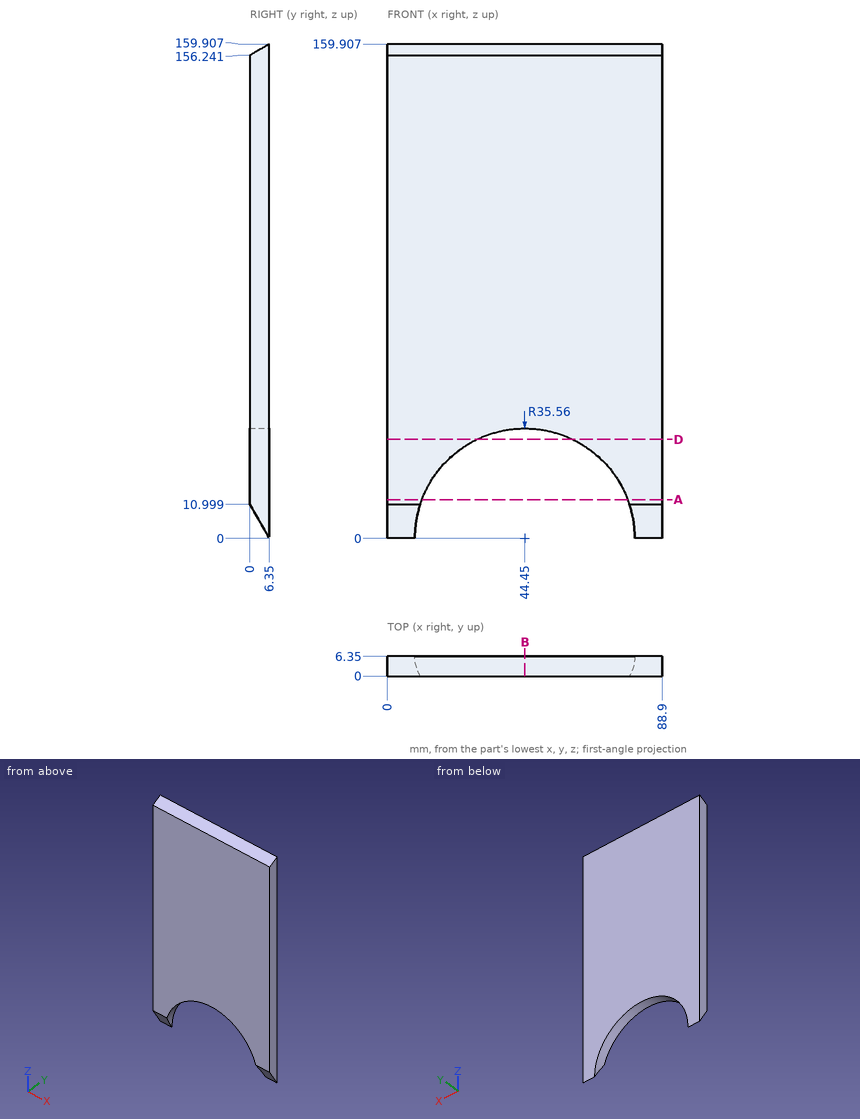
Verification items for this drawing (mm, ordinates from the low corner). Give positions to 0.01 mm unless a question says otherwise; leave off trailing zeros. Loops run counter-clockwise (first coordinate to the right, second up) from the corner with the lowest first, then second, coordinate; pieces in that order, holes last. Notation, with made-up numbers: M 39.5,41.25 L 43.5,41.25 A17 ccw 43.5,65.25 Z; hole C 0.5,12 d4. An arc over 180 degrees is marked long. Answer as a JSON object with one key per item and string values. Group by question number.
Q1. Cross-section at D-D on z = 32. Record the cut outline in (x, y).
Q2. Material ranges on line 1 along X through (y, z) = (3, 29); line 2 along X through (y, z) = (3, 29.5) (1 decimal); line 3 along Z through (x, y) = (65, 5.75), recorded low to high. Write a range as [from, to].
Q3. Go/stop test with flat-tipped pins: P1, Ø2, axis at x = 70, y = 4, coming from the +Z side; P2, Ø3, axis at x = 29, y = 4.5, coming from the +Z side (1 decimal); P3, Ø2, axis at x = 32, y = 5, coming from the -Z side; P4, Ø5, axis at x = 28.5, z = 29, coming from the +Y side. Record where each tip stops, or that it passes through.
Q4. Cross-section at B-B on x = 44.45. Record the cut outline in (y, z).
Q5. Cross-section at A-A on z = 12.5. Record the cut outline in (x, y).
Evaluation:
{
 "1": {"outline": "M 0,0 L 28.94,0 L 28.94,6.35 L 0,6.35 Z; M 59.96,0 L 88.9,0 L 88.9,6.35 L 59.96,6.35 Z"},
 "2": {"line 1": "x = [0, 23.87], [65.03, 88.9]", "line 2": "x = [0, 24.6], [64.3, 88.9]", "line 3": "z = [29.02, 159.56]"},
 "3": {"P1": "stops at z = 159.13", "P2": "stops at z = 159.7", "P3": "stops at z = 32.92", "P4": "stops at y = 6.35"},
 "4": {"outline": "M 0,35.56 L 6.35,35.56 L 6.35,159.91 L 0,156.24 Z"},
 "5": {"outline": "M 0,0 L 11.16,0 L 11.16,6.35 L 0,6.35 Z; M 77.74,0 L 88.9,0 L 88.9,6.35 L 77.74,6.35 Z"}
}
